Design review of the part built by this model. Coordinates are the model's own, in mm. Face numbers are marked on the shaded views. A direction names the side the tool comes from. Coordinates: 2 decimals unless noted, no trailing zeros. Write each loop counter-clockwise with the first axis right and the second up, starting at its lowest first coordinate (ties: lowest second). Pieces come first, ordered by that corner, then holes.
Q1. Take a section at A-A (y = 44). Give the boundary of the cut face in (x, z).
Q2. Machinability: for the marked faces 1 and 2, which of the approach directions +Z, -Z, +X, -X, +Y, -Y give a long, thin tool a straight path to every point of the face, cutting with its end or side? Answer none if there is none.
Q3. Insertion check: pin 1 (3.5 mm diameter, centred on x = 5, z = 2.5, fed in from +Y); pin 2 (0.9 mm diameter, centred on x = 34.5, z = 3, fed in from +Y). Each pin has a flat end and moves straight along its axis. Give the tip position at first contact, or say it passes through.
Q4. Take a section at B-B (x = 20). Give the boundary of the cut face in (y, z).
Q5. For probe 1 along X at (y, z) = (13, 1.95); probe 2 along X at (y, z) = (40, 1.5); probe 3 along Y at (x, z) = (26, 1.1), list the stretches that pass through material, from the lowest coordinate up.
Q6. Mouldability with a two-part tool opening along X and no side actions: class the marked faces 3, 4 and 5 as pulls with the +X half, pulls with the -X half, needs draft (parallel to the pull), parting line crosses it, or undercut.
Q7. Take a section at D-D (x = 12). Give the boundary of the cut face in (y, z), and give its area (3 significant figures).
Autodesk Fusion 360 part; units mm, degrees
sketch "Sketch1" plane through (0, 0, 0) normal (0, 0, 1) x (1, 0, 0)
  line L0 (0, 0) -> (40, 0)
  line L1 (40, 0) -> (40, 60)
  line L2 (40, 60) -> (0, 60)
  line L3 (0, 60) -> (0, 0)
  line L4 (20, 60) -> (20, 27.089)
  circle A0 centre (20, 40) radius 5
  line L5 (6.5, 0) -> (13.5, 0)
  line L6 (13.5, 0) -> (13.5, 25)
  line L7 (13.5, 25) -> (6.5, 25)
  line L8 (6.5, 25) -> (6.5, 0)
  line L9 (26.5, 0) -> (33.5, 0)
  line L10 (33.5, 0) -> (33.5, 25)
  line L11 (33.5, 25) -> (26.5, 25)
  line L12 (26.5, 25) -> (26.5, 0)
  line L13 (10, 25) -> (30, 25)
  line L14 (20, 25) -> (20, 0)
  line L15 (0, 16) -> (40, 16)
  line L16 (3.5, 16) -> (16.5, 16)
  line L17 (16.5, 16) -> (16.5, 9)
  line L18 (16.5, 9) -> (3.5, 9)
  line L19 (3.5, 9) -> (3.5, 16)
  line L20 (3.5, 12.5) -> (6.5, 12.5)
  line L21 (10, 9) -> (10, 0)
  line L22 (23.5, 16) -> (23.5, 9)
  line L23 (23.5, 9) -> (36.5, 9)
  line L24 (36.5, 9) -> (36.5, 16)
  dimension "d1" = 40
  dimension "d2" = 60
  dimension "d3" = 10
  dimension "d4" = 40
  dimension "d5" = 7
  dimension "d6" = 7
  dimension "d7" = 25
  dimension "d8" = 25
  dimension "d9" = 20
  dimension "d10" = 90
  dimension "d11" = 90
  dimension "d12" = 13
  dimension "d13" = 90
  dimension "d14" = 7
extrude "Extrude1" add sketch "Sketch1" along normal blind 6 contours L0 L3 L8 L15 L18 L19 | L1 L2 L3 L7 L8 L10 L11 L13 L15 L16 | L0 L6 L14 L15 L17 L18 | L0 L12 L14 L15 L22 L23 | L6 L13 L14 L15 L16 | L12 L13 L14 L15 | L0 L1 L10 L15 L23 L24
fillet "Fillet1" radius 10 1 edges at (0, 60, 3)
fillet "Fillet2" radius 10 1 edges at (40, 60, 3)
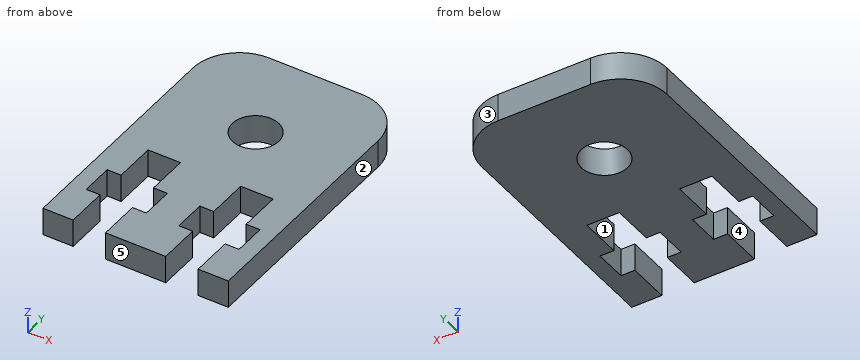
Response:
1. outline: (0, 0) - (17, 0) - (17, 6) - (0, 6) - close; (23, 0) - (40, 0) - (40, 6) - (23, 6) - close
2. face 1: +Z, -Z, -Y
2. face 2: +Z, -Z, +X, +Y, -Y
3. pin 1: stops at y = 59.46
3. pin 2: stops at y = 59.14
4. outline: (0, 0) - (35, 0) - (35, 6) - (0, 6) - close; (45, 0) - (60, 0) - (60, 6) - (45, 6) - close
5. probe 1: x = 0 to 3.5, 16.5 to 23.5, 36.5 to 40
5. probe 2: x = 0 to 15, 25 to 40
5. probe 3: y = 0 to 9, 16 to 60
6. face 3: pulls with the +X half
6. face 4: undercut
6. face 5: needs draft
7. outline: (25, 0) - (60, 0) - (60, 6) - (25, 6) - close
7. area: 210 mm2
